```python
from build123d import *

# Parameters (mm, degrees)
SKETCH1_W                = 12.41
SKETCH1_H                = 23.75
BOSS_EXTRUDE1_DEPTH      = 22.71
SKETCH2_R                = 5.875
BOSS_EXTRUDE3_DEPTH      = 4.2
BOSS_EXTRUDE4_DEPTH      = 4
BOSS_EXTRUDE5_DEPTH      = 4.87
BOSS_EXTRUDE5_DEPTH_BACK = 27.62
SKETCH6_W                = 12.41
SKETCH6_H                = 2.46
SKETCH8_R                = 1.43
CUT_EXTRUDE1_DEPTH       = 36.929209565
SKETCH9_W                = 1.02
SKETCH9_H                = 2.455
CUT_EXTRUDE2_DEPTH       = 36.929209565
SKETCH10_R               = 2.45
SKETCH10_R_2             = 0.885
BOSS_EXTRUDE7_DEPTH      = 2.7
BOSS_EXTRUDE8_DEPTH      = 5
SKETCH13_R               = 2
BOSS_EXTRUDE9_DEPTH      = 4


with BuildPart() as part:
    # Sketch1 → Boss-Extrude1 (new body)
    with BuildSketch(Plane(origin=(0, 0, 0), x_dir=(1, 0, 0), z_dir=(0, 1, 0))):
        with Locations((6.205, 11.875)):
            Rectangle(SKETCH1_W, SKETCH1_H)
    extrude(amount=BOSS_EXTRUDE1_DEPTH)

    # Sketch2 → Boss-Extrude3 (add)
    with BuildSketch(Plane.XY):
        with Locations(Location((6.205, 5.875, 0), (0, 0, 270))):
            Circle(SKETCH2_R)
    extrude(amount=BOSS_EXTRUDE3_DEPTH)

    # Sketch4 → Boss-Extrude4 (add)
    with BuildSketch(Plane.XY):
        with BuildLine():
            Line((3.43, 11.965), (3.43, 11.053320191))
            Line((3.43, 11.053320191), (8.98, 11.053320191))
            Line((8.98, 11.053320191), (8.98, 11.965))
            ThreePointArc((8.98, 11.965), (6.205, 14.74), (3.43, 11.965))
        make_face()
    extrude(amount=BOSS_EXTRUDE4_DEPTH)

    # Sketch6 → Boss-Extrude5 (add, two sides: drawn at the far end of the back side and taken through both)
    with BuildSketch(Plane.XZ.offset(-BOSS_EXTRUDE5_DEPTH_BACK)):
        with Locations((6.205, -5.64)):
            Rectangle(SKETCH6_W, SKETCH6_H)
    extrude(amount=BOSS_EXTRUDE5_DEPTH + BOSS_EXTRUDE5_DEPTH_BACK)

    # Sketch8 → Cut-Extrude1 (cut, through all)
    with BuildSketch(Plane.XY.offset(-4.41)):
        with Locations((6.205, 25.165)):
            Circle(SKETCH8_R)
        with Locations((6.205, -2.415)):
            Circle(SKETCH8_R)
    extrude(amount=-CUT_EXTRUDE1_DEPTH, mode=Mode.SUBTRACT)

    # Sketch9 → Cut-Extrude2 (cut, through all)
    with BuildSketch(Plane.XY.offset(-4.41)):
        with Locations((6.205, 26.3925)):
            Rectangle(SKETCH9_W, SKETCH9_H)
        with Locations((6.205, -3.6425)):
            Rectangle(SKETCH9_W, SKETCH9_H)
    extrude(amount=-CUT_EXTRUDE2_DEPTH, mode=Mode.SUBTRACT)

    # Sketch10 → Boss-Extrude7 (add)
    with BuildSketch(Plane.XY.offset(4.2)):
        with Locations(Location((6.205, 5.875, 0), (0, 0, 180))):
            Circle(SKETCH10_R)
        with Locations(Location((6.205, 5.875, 0), (0, 0, 180))):
            Circle(SKETCH10_R_2, mode=Mode.SUBTRACT)
    extrude(amount=BOSS_EXTRUDE7_DEPTH)

    # Sketch12 → Boss-Extrude8 (add)
    with BuildSketch(Plane.XZ):
        with BuildLine():
            ThreePointArc((5.61, -22.289411255), (6.205, -22.635), (6.8, -22.289411255))
            ThreePointArc((6.8, -22.289411255), (8.08, -21.95), (6.8, -21.610588745))
            ThreePointArc((6.8, -21.610588745), (6.205, -21.265), (5.61, -21.610588745))
            ThreePointArc((5.61, -21.610588745), (4.33, -21.95), (5.61, -22.289411255))
        make_face()
    extrude(amount=BOSS_EXTRUDE8_DEPTH)

    # Sketch13 → Boss-Extrude9 (add)
    with BuildSketch(Plane.XY.offset(6.9)):
        with Locations((6.205, 5.875)):
            Circle(SKETCH13_R)
    extrude(amount=BOSS_EXTRUDE9_DEPTH)


solid = part.part
```
The model under review builds one solid part; all positions refer to its coordinate system, in mm. A direction names the side the tool comes from. Round coordinates to 2 decimals unless told otherwise and drop trailing zeros. Order: outer loops, then holes, each group sorted by start corner. A loop starts at its lowest first (then second) coordinate and runs counter-clockwise, first axis right, second up. Notation, with made-up numbers: (52, 17) -> (75, 17) arc R25 cw to (75, 51) -> close; hole circle Ø7 at (68, 50). An arc over 180 degrees is marked (long way). One line per item, written item: value. Start each with the question number.
Q1. Take a section at C-C (x = 1.25). Write out the cut boundary in (y, z), and give its area (3 significant figures).
Q2. Machinability: for faces 1 (the face through (4.7, 25.7, -6.87)), 2 (the face through (6, 22.71, -2)), 3 (the face through (6, 0, -2)), 4 (the face through (4.7, -1.9, -6.87)), 5 (the face through (7.09, 5.84, 5.53)), which of the approach directions +Z, -Z, +X, -X, +Y, -Y give a long, thin tool a straight path to every point of the face, cutting with its end or side? Answer none if there is none.
Q3. Clearance check with flat-ended pins moving along their axes: pin 1 Ø4 at (x, y) = (8, 24.5) entering from +Z; pin 2 Ø2.5 at (x, y) = (4, 24.5) entering from -Z; pin 3 Ø1.5 at (x, y) = (9, 2.5) entering from +Z; pin 4 Ø10 at (y, z) = (14, 3) entering from -X. State where each tip first meets the part, or that it passes through.
Q4. Take a section at D-D (y = 13). Write out the cut boundary in (x, z).
Q5. Take a section at A-A (z = -11). Write out the cut boundary in (x, y), and give its area (3 significant figures).
Q6. Take a section at B-B (y = 3). Write out the cut boundary in (x, z).
Q7. Wall thickness on line 1 (Y direction, x = 6.75, z = -5); line 2 (Z direction, x = 6.75, y = 10); line 3 (Y direction, x = 7.25, z = -21.5): over which ranges is each line inside the solid? List them lowest first.
Q8. Mouldability with a two-part tool opening along Y and no side actions: class faces 6 (the face through (6, -1, -6)), 7 (the face through (6, 6, 6.9)), 8 (the face through (7, 8, 6.9)), 9 (the face through (3, -4.87, -6)) as released by +Y, released by -Y, zero draft, split by the parting line, or undercut.
Reported:
1. outline: (-4.87, -6.87) -> (0, -6.87) -> (0, -23.75) -> (22.71, -23.75) -> (22.71, -6.87) -> (27.62, -6.87) -> (27.62, -4.41) -> (22.71, -4.41) -> (22.71, 0) -> (9.03, 0) -> (9.03, 4.2) -> (2.72, 4.2) -> (2.72, 0) -> (0, 0) -> (0, -4.41) -> (-4.87, -4.41) -> close
1. area: 590 mm2
2. face 1: -Z, +X, -X, +Y
2. face 2: +Z, +X, -X, +Y
2. face 3: +Z, +X, -X, -Y
2. face 4: +X, -X, -Y
2. face 5: none
3. pin 1: stops at z = 0
3. pin 2: stops at z = -6.87
3. pin 3: stops at z = 4.2
3. pin 4: stops at x = 0
4. outline: (0, -23.75) -> (12.41, -23.75) -> (12.41, 0) -> (8.78, 0) -> (8.78, 4) -> (3.63, 4) -> (3.63, 0) -> (0, 0) -> close
5. outline: (0, 0) -> (12.41, 0) -> (12.41, 22.71) -> (0, 22.71) -> close
5. area: 282 mm2
6. outline: (0, -23.75) -> (12.41, -23.75) -> (12.41, 0) -> (11.33, 0) -> (11.33, 4.2) -> (1.08, 4.2) -> (1.08, 0) -> (0, 0) -> close
7. line 1: y = -4.87 to -3.74, -1.09 to 23.84, 26.49 to 27.62
7. line 2: z = -23.75 to 4.2
7. line 3: y = -5 to 22.71
8. face 6: undercut
8. face 7: undercut
8. face 8: zero draft
8. face 9: released by -Y
